Model file for the job. Use its own axes, mm. A direction names the side the tool comes from. Give positions to 0.01 mm unless a question says otherwise; leave off trailing zeros. Order: outer loops, then holes, each group sorted by start corner. A loop starts at its lowest first (then second) coordinate and runs counter-clockwise, first axis right, second up. Notation, with made-up numbers: (-6.5, 74.25) - (4.5, 74.25) arc R14 cw to (4.5, 88.25) - close; hole circle Ø7 at (11.25, 61.5). An arc over 180 degrees is marked (long way). Return JSON: item names as keys, results as strings. Group by question number.
from build123d import *

# Parameters (mm, degrees)
SKETCH_1_R          = 55
EXTRUDE_1_DEPTH     = 9
SKETCH_2_R          = 30.95
EXTRUDE_2_DEPTH     = 21.96
SKETCH_3_R          = 27
CUT_EXTRUDE_1_DEPTH = 18.5
CUT_EXTRUDE_1_TAPER = 2
FILLET_1_R          = 3
SKETCH_4_R          = 14
CUT_EXTRUDE_2_DEPTH = 18.5
SKETCH_5_W          = 3
SKETCH_5_H          = 6
SKETCH_7_R          = 32
CUT_EXTRUDE_3_DEPTH = 1
CUT_EXTRUDE_4_DEPTH = 20


with BuildPart() as part:
    # 草图1 → 凸台-拉伸1 (new body)
    with BuildSketch(Plane(origin=(0, 0, 0), x_dir=(0, 0, -1), z_dir=(1, 0, 0))):
        Circle(SKETCH_1_R)
    extrude(amount=EXTRUDE_1_DEPTH)

    # 草图2 → 凸台-拉伸2 (add)
    with BuildSketch(Plane(origin=(9, 0, 0), x_dir=(0, 0, -1), z_dir=(1, 0, 0))):
        Circle(SKETCH_2_R)
    extrude(amount=EXTRUDE_2_DEPTH)

    # 草图3 → 切除-拉伸1 (cut)
    with BuildSketch(Plane(origin=(30.96, 0, 0), x_dir=(0, 0, -1), z_dir=(1, 0, 0))):
        Circle(SKETCH_3_R)
    extrude(amount=-CUT_EXTRUDE_1_DEPTH, taper=CUT_EXTRUDE_1_TAPER, mode=Mode.SUBTRACT)

    # 圆角1
    fillet_1_edges = [part.edges().sort_by_distance(p)[0] for p in [
        (12.46, 0, 26.353965764),
    ]]
    fillet(fillet_1_edges, radius=FILLET_1_R)

    # 草图4 → 切除-拉伸2 (cut)
    with BuildSketch(Plane(origin=(12.46, 0, 0), x_dir=(0, 0, -1), z_dir=(1, 0, 0))):
        Circle(SKETCH_4_R)
    extrude(amount=-CUT_EXTRUDE_2_DEPTH, mode=Mode.SUBTRACT)

    # 切除-扫描1: sweep along a path in 草图6
    with BuildLine(Plane(origin=(4.5, 0, 14), x_dir=(0, 0, -1), z_dir=(1, 0, 0))) as sweep_1_path:
        CenterArc((14, 0), 14, 0, 360)
    # 草图5 → 切除-扫描1 (sweep, cut)
    with BuildSketch(Plane(origin=(0, 0, 0), x_dir=(1, 0, 0), z_dir=(0, 1, 0))):
        with Locations((4.5, -14)):
            Rectangle(SKETCH_5_W, SKETCH_5_H)
    sweep(path=sweep_1_path.line, mode=Mode.SUBTRACT)

    # 草图7 → 切除-拉伸3 (cut)
    with BuildSketch(Plane.ZY):
        Circle(SKETCH_7_R)
    extrude(amount=-CUT_EXTRUDE_3_DEPTH, mode=Mode.SUBTRACT)

    # 草图8 → 切除-拉伸4 (cut)
    with BuildSketch(Plane.ZY):
        with BuildLine():
            ThreePointArc((0, 47.5), (-4, 43.5), (0, 39.5))
            Line((0, 39.5), (0, 47.5))
        make_face()
        with BuildLine():
            Line((0, 47.5), (0, 39.5))
            ThreePointArc((0, 39.5), (2.828427125, 40.671572875), (4, 43.5))
            ThreePointArc((4, 43.5), (2.828427125, 46.328427125), (0, 47.5))
        make_face()
        with BuildLine():
            ThreePointArc((47.5, 0), (43.5, 4), (39.5, 0))
            Line((39.5, 0), (47.5, 0))
        make_face()
        with BuildLine():
            Line((47.5, 0), (39.5, 0))
            ThreePointArc((39.5, 0), (43.5, -4), (47.5, 0))
        make_face()
        with BuildLine():
            ThreePointArc((0, -39.5), (-4, -43.5), (0, -47.5))
            Line((0, -47.5), (0, -39.5))
        make_face()
        with BuildLine():
            Line((0, -39.5), (0, -47.5))
            ThreePointArc((0, -47.5), (2.828427125, -46.328427125), (4, -43.5))
            ThreePointArc((4, -43.5), (2.828427125, -40.671572875), (0, -39.5))
        make_face()
        with BuildLine():
            ThreePointArc((-39.5, 0), (-43.5, 4), (-47.5, 0))
            Line((-47.5, 0), (-39.5, 0))
        make_face()
        with BuildLine():
            Line((-39.5, 0), (-47.5, 0))
            ThreePointArc((-47.5, 0), (-43.5, -4), (-39.5, 0))
        make_face()
    extrude(amount=-CUT_EXTRUDE_4_DEPTH, mode=Mode.SUBTRACT)


solid = part.part
(1) Slice it at C-C (y = 0). State how many separate pieces and enclosed holes the cut face has, and give its area (3 significant figures).
(2) Drop flat-ended pins along their axis: pin 1 Ø9 at (y, z) = (0, 43.5) entering from +X; pin 2 Ø25 at (y, z) = (0, 0) entering from -X; pin 3 Ø23.5 at (y, z) = (6.5, -3.5) entering from +X; pin 4 Ø6 at (x, z) = (4, 40.5) entering from -Y. Give the stop position or say it passes through.
(3) Pull direction Z, two halves, no side cores. Call faces 6 (the face through (2.014, -5.362, -12.932)), 7 (the face through (0, -24, -24)), 8 (the face through (19.826, -30.214, 6.709)): released by +Z, released by -Z, zero draft, split by the parting line, or undercut.
(4) Slice it at B-B (y = -45). Give the cut face in (x, z), and give its area (3 significant figures).
(5) Drill centre lines: L1, parallel to Y at x = 0.65, z = 0; L2, parallel to X at y = 12, z = 16.5; L3, parallel to Z at x = 28.5, y = 12. Where is each one in solid material? Low to high.
(6) Slice it at A-A (z = 43.5). Give the cut face in (x, y), and give its area (3 significant figures).
(7) Slice it at D-D (x = 26). Give the cut face in (y, z).
(8) 3-axis set-ups, long thin cutter, end or side, ignore diameter. For faces 1 (the face through (30.96, 28, -2)), 2 (the face through (4.521, 5.106, -16.215)), 3 (the face through (4.4, 2.4, 46.7)), 4 (the face through (9, -24, -24)), 5 (the face through (0.49, -31.24, -6.94)): which of +Z, -Z, +X, -X, +Y, -Y reach the whole face in a straight line?
Result set:
{
 "1": {"separate pieces": "4", "enclosed holes": "0", "area": "819 mm²"},
 "2": {"pin 1": "stops at x = 9", "pin 2": "passes through", "pin 3": "stops at x = 12.46", "pin 4": "stops at y = -40.23"},
 "3": {"face 6": "undercut", "face 7": "zero draft", "face 8": "split by the parting line"},
 "4": {"outline": "(0, -31.62) - (9, -31.62) - (9, -3.71) - (0, -3.71) - close; (0, 3.71) - (9, 3.71) - (9, 31.62) - (0, 31.62) - close", "area": "502 mm²"},
 "5": {"L1": "y = -55 to -47.5, -39.5 to -32, 32 to 39.5, 47.5 to 55", "L2": "x = 1 to 12.46", "L3": "z = -28.53 to -24.09, 24.09 to 28.53"},
 "6": {"outline": "(0, -33.66) - (9, -33.66) - (9, -4) - (0, -4) - close; (0, 4) - (9, 4) - (9, 33.66) - (0, 33.66) - close", "area": "534 mm²"},
 "7": {"outline": "circle Ø61.9 at (0, 0); hole circle Ø53.65 at (0, 0)"},
 "8": {"face 1": "+Z, -Z, +X, +Y, -Y", "face 2": "none", "face 3": "+X, -X", "face 4": "+X", "face 5": "-X"}
}
